```python
from build123d import *

# Parameters (mm, degrees)
EXTRUDE_1_DEPTH     = 1
EXTRUDE_2_DEPTH     = 4.5
SKETCH_4_R          = 2
EXTRUDE_3_DEPTH     = 2.5
CHAMFER_1_SIZE      = 1
EXTRUDE_4_OUTLINE_R = 2
EXTRUDE_4_DEPTH     = 1.5
SKETCH_6_R          = 1
CUT_EXTRUDE_1_DEPTH = 115.249760713


# Read off the part's stored shape, not the designer's step: Бобышка-Вытянуть4
with BuildPart() as part:
    # Эскиз2 → Бобышка-Вытянуть1 (new body)
    with BuildSketch(Plane.XY):
        with BuildLine():
            Line((2.50000008, 78.20000148), (68.99999916, 78.19999894))
            ThreePointArc((68.99999916, 78.19999894), (70.909187526, 77.409187226), (71.69999924, 75.49999886))
            Line((71.69999924, 75.49999886), (71.70000051, 2.500002823))
            ThreePointArc((71.70000051, 2.500002823), (70.909189394, 0.590811786), (68.99999916, -0.20000127))
            Line((68.99999916, -0.20000127), (2.50000008, -0.20000127))
            ThreePointArc((2.50000008, -0.20000127), (0.590809846, 0.590811786), (-0.20000127, 2.500002823))
            Line((-0.20000127, 2.500002823), (-0.20000254, 75.49999886))
            ThreePointArc((-0.20000254, 75.49999886), (0.590809918, 77.409189022), (2.50000008, 78.20000148))
        make_face()
    extrude(amount=EXTRUDE_1_DEPTH)

    # Эскиз3 → Бобышка-Вытянуть2 (add)
    with BuildSketch(Plane.XY):
        with BuildLine():
            Line((-1.20000254, 75.49999886), (-1.20000127, 2.500002806))
            ThreePointArc((-1.20000127, 2.500002806), (-0.116296929, -0.116295001), (2.50000008, -1.20000127))
            Line((2.50000008, -1.20000127), (68.99999916, -1.20000127))
            ThreePointArc((68.99999916, -1.20000127), (71.616296534, -0.116294636), (72.70000051, 2.500003839))
            Line((72.70000051, 2.500003839), (72.69999924, 75.499998877))
            ThreePointArc((72.69999924, 75.499998877), (71.616294301, 78.116294013), (68.99999916, 79.19999894))
            Line((68.99999916, 79.19999894), (2.50000008, 79.20000148))
            ThreePointArc((2.50000008, 79.20000148), (-0.116296863, 78.116295803), (-1.20000254, 75.49999886))
        make_face()
        with BuildLine():
            Line((-0.20000254, 75.49999886), (-0.20000127, 2.500002823))
            ThreePointArc((-0.20000127, 2.500002823), (0.590809846, 0.590811786), (2.50000008, -0.20000127))
            Line((2.50000008, -0.20000127), (68.99999916, -0.20000127))
            ThreePointArc((68.99999916, -0.20000127), (70.909189394, 0.590811786), (71.70000051, 2.500002823))
            Line((71.70000051, 2.500002823), (71.69999924, 75.49999886))
            ThreePointArc((71.69999924, 75.49999886), (70.909187526, 77.409187226), (68.99999916, 78.19999894))
            Line((68.99999916, 78.19999894), (2.50000008, 78.20000148))
            ThreePointArc((2.50000008, 78.20000148), (0.590809918, 77.409189022), (-0.20000254, 75.49999886))
        make_face(mode=Mode.SUBTRACT)
    extrude(amount=EXTRUDE_2_DEPTH)


with BuildPart() as extrude_3_tool:
    # Эскиз4 → Бобышка-Вытянуть3 (new body)
    # profile 1 of 2: a face of its own
    with BuildSketch(Plane.XY):
        with BuildLine():
            Line((-6.805028483, 42.99999886), (-1.200001975, 42.99999886))
            Line((-1.200001975, 42.99999886), (-1.200001835, 34.99999886))
            Line((-1.200001835, 34.99999886), (-6.805028483, 34.99999886))
            ThreePointArc((-6.805028483, 34.99999886), (-10.805028483, 38.99999886), (-6.805028483, 42.99999886))
        make_face()
        with Locations((-6.805028483, 38.99999886)):
            Circle(SKETCH_4_R, mode=Mode.SUBTRACT)
    # profile 2 of 2: a face of its own
    with BuildSketch(Plane.XY):
        with BuildLine():
            Line((72.700001075, 34.99999886), (78.305027723, 34.99999886))
            ThreePointArc((78.305027723, 34.99999886), (82.305027723, 38.99999886), (78.305027723, 42.99999886))
            Line((78.305027723, 42.99999886), (72.700001215, 42.99999886))
            Line((72.700001215, 42.99999886), (72.700001075, 34.99999886))
        make_face()
        with Locations(Location((78.305027723, 38.99999886, 0), (0, 0, 180))):
            Circle(SKETCH_4_R, mode=Mode.SUBTRACT)
    extrude(amount=EXTRUDE_3_DEPTH)


with BuildPart() as part_1:
    add(part.part)


with BuildPart() as part_2:
    # Бобышка-Вытянуть3: joined with extrude_3_tool
    add(part_1.part.fuse(extrude_3_tool.part, tol=0.00001))

    # Фаска1
    chamfer_1_edges = [part_2.edges().sort_by_distance(p)[0] for p in [
        (-8.805028483, 38.99999886, 2.5),
        (80.305027723, 38.99999886, 2.5),
    ]]
    chamfer(chamfer_1_edges, length=CHAMFER_1_SIZE)

    # Бобышка-Вытянуть4 outline → Бобышка-Вытянуть4 (add)
    with BuildSketch(Plane.XY.offset(1)):
        with BuildLine():
            Line((68.14600291, 39.521136107), (71.699999866, 39.521136107))
            Line((71.699999866, 39.521136107), (71.699999782, 44.345437587))
            Line((71.699999782, 44.345437587), (68.14600291, 44.345437587))
            ThreePointArc((68.14600291, 44.345437587), (66.731789347, 43.75965115), (66.14600291, 42.345437587))
            Line((66.14600291, 42.345437587), (66.14600291, 41.521136107))
            ThreePointArc((66.14600291, 41.521136107), (66.731789347, 40.106922544), (68.14600291, 39.521136107))
        make_face()
        with BuildLine():
            Line((66.497946234, 2.977437415), (66.497946234, -0.20000127))
            Line((66.497946234, -0.20000127), (68.99999916, -0.20000127))
            ThreePointArc((68.99999916, -0.20000127), (70.909189394, 0.590811786), (71.70000051, 2.500002823))
            Line((71.70000051, 2.500002823), (71.700000467, 4.977437415))
            Line((71.700000467, 4.977437415), (68.497946234, 4.977437415))
            ThreePointArc((68.497946234, 4.977437415), (67.083732671, 4.391650978), (66.497946234, 2.977437415))
        make_face()
        with BuildLine():
            Line((54.934013046, 78.199999477), (49.186165717, 78.199999697))
            Line((49.186165717, 78.199999697), (49.186165717, 74.793776217))
            ThreePointArc((49.186165717, 74.793776217), (49.771952154, 73.379562654), (51.186165717, 72.793776217))
            Line((51.186165717, 72.793776217), (52.934013046, 72.793776217))
            ThreePointArc((52.934013046, 72.793776217), (54.348226608, 73.379562655), (54.934013046, 74.793776217))
            Line((54.934013046, 74.793776217), (54.934013046, 78.199999477))
        make_face()
        with BuildLine():
            Line((-0.20000254, 75.49999886), (-0.200002499, 73.133544525))
            Line((-0.200002499, 73.133544525), (3.577150519, 73.133544525))
            ThreePointArc((3.577150519, 73.133544525), (4.991364081, 73.719330963), (5.577150519, 75.133544525))
            Line((5.577150519, 75.133544525), (5.577150519, 78.200001362))
            Line((5.577150519, 78.200001362), (2.50000008, 78.20000148))
            ThreePointArc((2.50000008, 78.20000148), (0.590809918, 77.409189022), (-0.20000254, 75.49999886))
        make_face()
        with BuildLine():
            Line((-0.200002102, 50.30535038), (-0.200001905, 39.000000842))
            Line((-0.200001905, 39.000000842), (3.837355963, 39.000000842))
            ThreePointArc((3.837355963, 39.000000842), (5.251569526, 39.585787279), (5.837355963, 41.000000842))
            Line((5.837355963, 41.000000842), (5.837355963, 48.30535038))
            ThreePointArc((5.837355963, 48.30535038), (5.251569526, 49.719563943), (3.837355963, 50.30535038))
            Line((3.837355963, 50.30535038), (-0.200002102, 50.30535038))
        make_face()
        with BuildLine():
            ThreePointArc((5.080506282, 2.977437415), (4.494719845, 4.391650977), (3.080506282, 4.977437415))
            Line((3.080506282, 4.977437415), (-0.200001313, 4.977437415))
            Line((-0.200001313, 4.977437415), (-0.20000127, 2.500002823))
            ThreePointArc((-0.20000127, 2.500002823), (0.590809846, 0.590811786), (2.50000008, -0.20000127))
            Line((2.50000008, -0.20000127), (5.080506282, -0.20000127))
            Line((5.080506282, -0.20000127), (5.080506282, 2.977437415))
        make_face()
        with Locations((52.00000014, 47.49999898)):
            Circle(EXTRUDE_4_OUTLINE_R)
    extrude(amount=EXTRUDE_4_DEPTH)

    # Эскиз6 → Вырез-Вытянуть1 (cut, through all)
    with BuildSketch(Plane.XY.offset(2.5)):
        with Locations((52.00000014, 75.49999886)):
            Circle(SKETCH_6_R)
        with Locations((2.99999908, 75.49999886)):
            Circle(SKETCH_6_R)
        with Locations((2.99999908, 47.49999898)):
            Circle(SKETCH_6_R)
        with Locations((2.50000008, 41.99999982)):
            Circle(SKETCH_6_R)
        with Locations((2.50000008, 2.50000008)):
            Circle(SKETCH_6_R)
        with Locations((68.99999916, 2.50000008)):
            Circle(SKETCH_6_R)
        with Locations((68.99999916, 41.99999982)):
            Circle(SKETCH_6_R)
        with Locations((52.00000014, 47.49999898)):
            Circle(SKETCH_6_R)
    extrude(amount=-CUT_EXTRUDE_1_DEPTH, mode=Mode.SUBTRACT)


solid = part_2.part
```
Part model, mm, in its own coordinate system. A direction names the side the tool comes from. Give positions to 0.01 mm unless a question says otherwise; leave off trailing zeros. Order: outer loops, then holes, each group sorted by start corner. A loop starts at its lowest first (then second) coordinate and runs counter-clockwise, first axis right, second up. Notation, with made-up numbers: M 15,51.25 L 24,51.25 A27 ccw 24,90.25 Z; hole C 45.25,15.25 d2. An arc over 180 degrees is marked long. Use a Markdown table: item, result. Add a question column.
(1) 3-axis set-ups, long thin cutter, end or side, ignore diameter. For faces 4 (the face through (69.924, 2.117, 1.268)), 5 (the face through (54.33, 73.36, 1.74)): which of +Z, -Z, +X, -X, +Y, -Y reach the whole face in a straight line?
(2) Drop flat-ended pins along their axis: P1, Ø1, axis at y = 46.5, z = 3.5, coming from the -X side; P2, Ø0.9, axis at y = 42, z = 2, coming from the -X side; P3, Ø2.5, axis at x = -8, y = 39, coming from the +Z side (3 decimals); P4, Ø1.6, axis at x = 69, y = 2.5, coming from the +Z side. Give the stop position or say it passes through.
(3) Mould opens along X. For faces 1 (the face through (4.51, 4.376, 1.74)), 2 (the face through (71.64, 78.09, 2.22)), 3 (the face through (-4, 41, 2.5)) say: +X half, -X half, draft (parallel to the pull), parting line (faces both ways), or undercut.
(4) Saw through at B-B, the plane z = 3.6. Give the cut face in (x, y), and give its area (3 significant figures).
(5) Probe line 1 along Y through (x, z) = (19, 3.9); line 2 along X through (y, z) = (6, 4.1); line 3 along X through (y, z) = (42, 1.75). List the from-to ranges inside material, lowest first. Write a range as [from, to].
(6) Saw through at C-C, the plane y = 18. Give the cut face in (x, z), and give its area (3 significant figures).
(7) Saw through at A-A, the plane x = 58.5. Give the cut face in (y, z), and give its area (3 significant figures).
Answer key:
| question | item | result |
|---|---|---|
| 1 | face 4 | +Z, -Z |
| 1 | face 5 | +Z |
| 2 | P1 | x = -1.2 |
| 2 | P2 | x = -9.89 |
| 2 | P3 | z = 1.945 |
| 2 | P4 | through |
| 3 | face 1 | undercut |
| 3 | face 2 | +X half |
| 3 | face 3 | draft |
| 4 | outline | M -1.2,2.5 A3.7 ccw 2.5,-1.2 L 69,-1.2 A3.7 ccw 72.7,2.5 L 72.7,75.5 A3.7 ccw 69,79.2 L 2.5,79.2 A3.7 ccw -1.2,75.5 Z; hole M -0.2,2.5 A2.7 ccw 2.5,-0.2 L 69,-0.2 A2.7 ccw 71.7,2.5 L 71.7,75.5 A2.7 ccw 69,78.2 L 2.5,78.2 A2.7 ccw -0.2,75.5 Z |
| 4 | area | 299 mm^2 |
| 5 | line 1 | [-1.2, -0.2], [78.2, 79.2] |
| 5 | line 2 | [-1.2, -0.2], [71.7, 72.7] |
| 5 | line 3 | [-9.45, 1.5], [3.5, 5.84], [66.15, 68], [70, 80.95] |
| 6 | outline | M -1.2,0 L 72.7,0 L 72.7,4.5 L 71.7,4.5 L 71.7,1 L -0.2,1 L -0.2,4.5 L -1.2,4.5 Z |
| 6 | area | 80.9 mm^2 |
| 7 | outline | M -1.2,0 L 79.2,0 L 79.2,4.5 L 78.2,4.5 L 78.2,1 L -0.2,1 L -0.2,4.5 L -1.2,4.5 Z |
| 7 | area | 87.4 mm^2 |
